Check sheet for the modelled part. Datum: model origin and axes. Units: mm. Round coordinates to 2 decimals unless told otherwise and drop trailing zeros. Loops run counter-clockwise (first coordinate to the right, second up) from the corner with the lowest first, then second, coordinate; pieces in that order, holes last. Notation, with made-up numbers: (-30.75, -25.75) -> (-4.75, -25.75) arc R3 ccw to (-4.75, -20.75) -> close; hole circle Ø10 at (-18.5, 27). An arc over 180 degrees is marked (long way). Use one line per item in the form item = value. Start each with the question number.
(1) Material ranges on probe 1 along Y at (x, z) = (22.5, 0.4); probe 2 along Y at (x, z) = (21, 0.85); probe 3 along Y at (x, z) = (-41, 0.85), recorded low to high. Write a range as [from, to].
(2) Go/stop test with a flat-tipped pin: pin 1 (1 mm diameter, centred on x = 16.5, y = 9, fed in from -Z). Record where the tip stops, or that it passes through.
(3) Sectioned sample at A-A (z = 0.25). Record the cut outline in (x, y), and give its area (3 significant figures).
(4) Sectioned sample at B-B (y = -37). Record the cut outline in (x, z), and give its area (3 significant figures).
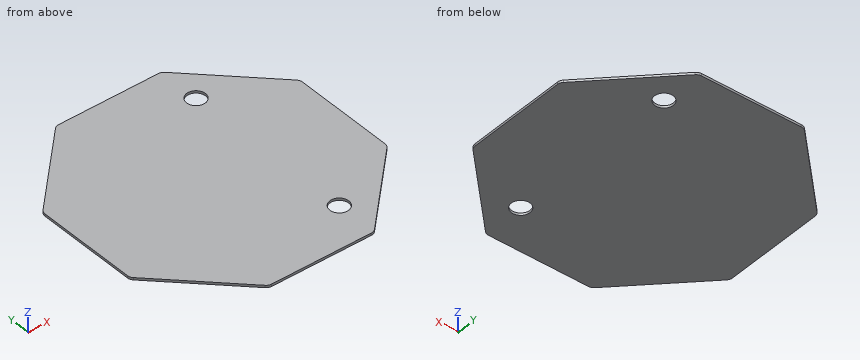
from build123d import *

# Parameters (mm, degrees)
SKETCH3_R           = 4
BOSS_EXTRUDE1_DEPTH = 1


with BuildPart() as part:
    # Sketch3 → Boss-Extrude1 (new body)
    with BuildSketch(Plane.XY):
        with BuildLine():
            Line((55, -21.257359313), (55, 21.257359313))
            ThreePointArc((55, 21.257359313), (54.771638598, 22.40540961), (54.121320344, 23.378679656))
            Line((54.121320344, 23.378679656), (23.378679656, 54.121320344))
            ThreePointArc((23.378679656, 54.121320344), (22.40540961, 54.771638598), (21.257359313, 55))
            Line((21.257359313, 55), (-21.257359313, 55))
            ThreePointArc((-21.257359313, 55), (-22.40540961, 54.771638598), (-23.378679656, 54.121320344))
            Line((-23.378679656, 54.121320344), (-54.121320344, 23.378679656))
            ThreePointArc((-54.121320344, 23.378679656), (-54.771638598, 22.40540961), (-55, 21.257359313))
            Line((-55, 21.257359313), (-55, -21.257359313))
            ThreePointArc((-55, -21.257359313), (-54.771638598, -22.40540961), (-54.121320344, -23.378679656))
            Line((-54.121320344, -23.378679656), (-23.378679656, -54.121320344))
            ThreePointArc((-23.378679656, -54.121320344), (-22.40540961, -54.771638598), (-21.257359313, -55))
            Line((-21.257359313, -55), (21.257359313, -55))
            ThreePointArc((21.257359313, -55), (22.40540961, -54.771638598), (23.378679656, -54.121320344))
            Line((23.378679656, -54.121320344), (54.121320344, -23.378679656))
            ThreePointArc((54.121320344, -23.378679656), (54.771638598, -22.40540961), (55, -21.257359313))
        make_face()
        with Locations((22.5, 37)):
            Circle(SKETCH3_R, mode=Mode.SUBTRACT)
        with Locations(Location((22.5, -37, 0), (0, 0, 180))):
            Circle(SKETCH3_R, mode=Mode.SUBTRACT)
    extrude(amount=BOSS_EXTRUDE1_DEPTH)


solid = part.part
Checks:
q1.probe_1 = [-54.73, -41], [-33, 33], [41, 54.73]
q1.probe_2 = [-55, -40.71], [-33.29, 33.29], [40.71, 55]
q1.probe_3 = [-36.5, 36.5]
q2.pin_1 = 0
q3.outline = (-55, -21.26) arc R3 ccw to (-54.12, -23.38) -> (-23.38, -54.12) arc R3 ccw to (-21.26, -55) -> (21.26, -55) arc R3 ccw to (23.38, -54.12) -> (54.12, -23.38) arc R3 ccw to (55, -21.26) -> (55, 21.26) arc R3 ccw to (54.12, 23.38) -> (23.38, 54.12) arc R3 ccw to (21.26, 55) -> (-21.26, 55) arc R3 ccw to (-23.38, 54.12) -> (-54.12, 23.38) arc R3 ccw to (-55, 21.26) -> close; hole circle Ø8 at (22.5, -37); hole circle Ø8 at (22.5, 37)
q3.area = 9,890 mm2
q4.outline = (-40.5, 0) -> (18.5, 0) -> (18.5, 1) -> (-40.5, 1) -> close; (26.5, 0) -> (40.5, 0) -> (40.5, 1) -> (26.5, 1) -> close
q4.area = 73.0 mm2
